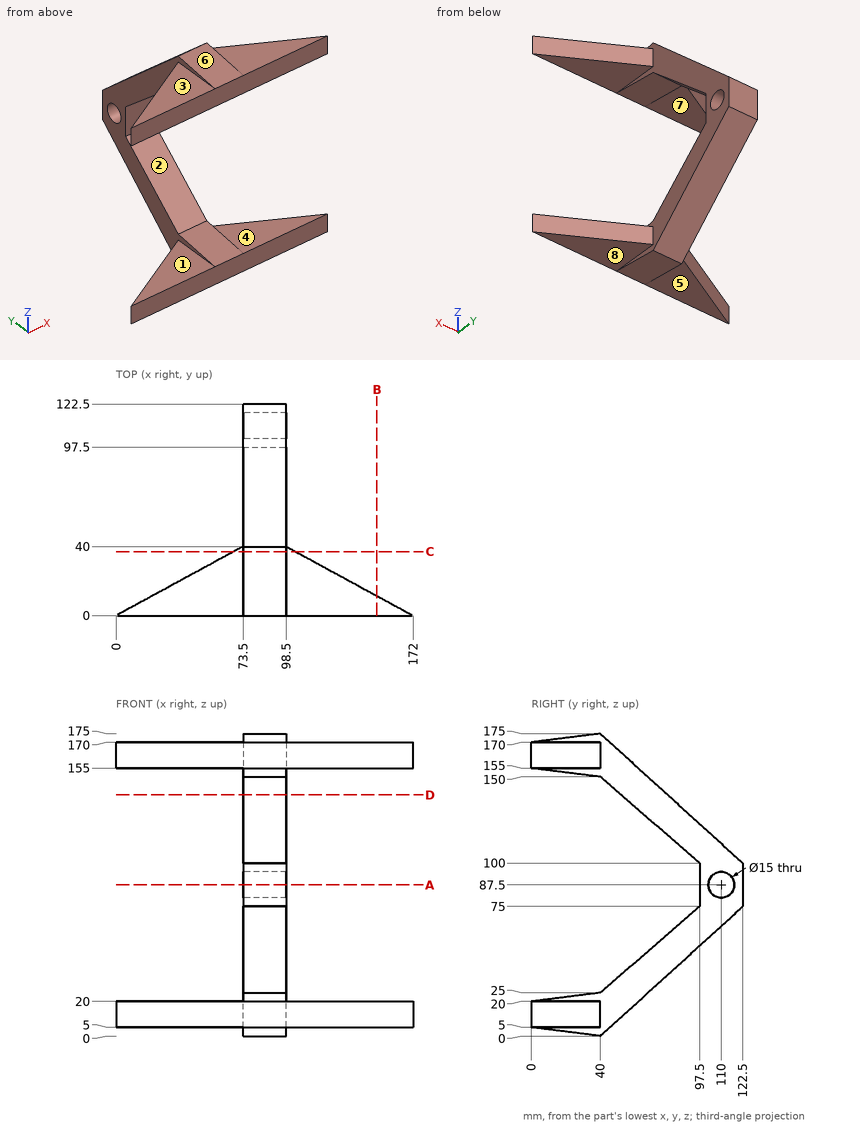
Here's the drawing with two shaded views (mm, measured from the low corner). I have some questions. A direction names the side the tool comes from. Coordinates: 2 decimals unless noted, no trailing zeros. Loops run counter-clockwise (first coordinate to the right, second up) from the corner with the lowest first, then second, coordinate; pieces in that order, holes last. Notation, with made-up numbers: (80.25, 8) -> (84.25, 8) arc R21 ccw to (84.25, 23) -> close; hole circle Ø3 at (-9.5, 39). An arc over 180 degrees is marked (long way). Put each result on its own line as item: value. Start each with the question number.
Q1. I want a section at A-A (z = 87.5). Write out the boundary of the cut face in (x, y).
Q2. I want a section at C-C (y = 37). Write out the boundary of the cut face in (x, z) (1 decimal).
Q3. I want a section at B-B (x = 151). Write out the boundary of the cut face in (y, z).
Q4. For the marked faces 1, 2, 3, 4 and 5, which set-ups out of +Z, -Z, +X, -X, +Y, -Y let a thin tool reach every point of the face, with its end or its side?
Q5. If I drill on line 1 (Y direction, x = 84, z = 87); line 2 (Z direction, x = 92, y = 110); line 3 (Z direction, x = 89, y = 71), over which ranges is the centre line in solid material (lowest first)? Write a range as [from, to].
Q6. I'm going to push flat-ended pins straight in: P1, Ø12, axis at x = 29.5, y = 22, coming from the -Z side; P2, Ø12, axis at x = 25, y = 18.5, coming from the +Z side; P3, Ø8, axis at x = 95, z = 108, coming from the -Y side. Where does each tip first touch, or does it pass through?
Q7. I want a section at D-D (z = 139.5). Write out the boundary of the cut face in (x, y) (3 decimals), plus the area to 3 significant figures.
Q8. Thinking about a two-plate mould opening in Z: for the marked faces 6, 7 and 8, which applies, pulls with the +Z half, pulls with the -Z half, needs draft (parallel to the pull), parting line crosses it, or undercut?
Taken from the geometry:
1. outline: (73.5, 97.5) -> (98.5, 97.5) -> (98.5, 102.5) -> (73.5, 102.5) -> close; (73.5, 117.5) -> (98.5, 117.5) -> (98.5, 122.5) -> (73.5, 122.5) -> close
2. outline: (68, 5) -> (73.5, 5) -> (73.5, 0.4) -> (98.5, 0.4) -> (98.5, 5) -> (104, 5) -> (104, 20) -> (98.5, 20) -> (98.5, 24.6) -> (73.5, 24.6) -> (73.5, 20) -> (68, 20) -> close; (68, 155) -> (73.5, 155) -> (73.5, 150.4) -> (98.5, 150.4) -> (98.5, 155) -> (104, 155) -> (104, 170) -> (98.5, 170) -> (98.5, 174.6) -> (73.5, 174.6) -> (73.5, 170) -> (68, 170) -> close
3. outline: (0, 5) -> (11.43, 5) -> (11.43, 20) -> (0, 20) -> close; (0, 155) -> (11.43, 155) -> (11.43, 170) -> (0, 170) -> close
4. face 1: -X, +Y, -Y
4. face 2: +X, -X, -Y
4. face 3: +Z, -X, +Y, -Y
4. face 4: +X, +Y, -Y
4. face 5: -Z, -X, +Y, -Y
5. line 1: y = [97.5, 102.52], [117.48, 122.5]
5. line 2: z = [63.64, 80], [95, 111.36]
5. line 3: z = [28.18, 51.96], [123.04, 146.82]
6. P1: stops at z = 5
6. P2: stops at z = 170
6. P3: stops at y = 83.7
7. outline: (73.5, 52.075) -> (98.5, 52.075) -> (98.5, 79.05) -> (73.5, 79.05) -> close
7. area: 674 mm2
8. face 6: pulls with the +Z half
8. face 7: undercut
8. face 8: pulls with the -Z half
